Geometry check sheet. Reference: the model listing, model coordinates, mm. A direction names the side the tool comes from. Round coordinates to 2 decimals unless told otherwise and drop trailing zeros. Loops run counter-clockwise (first coordinate to the right, second up) from the corner with the lowest first, then second, coordinate; pieces in that order, holes last. Notation, with made-up numbers: (50.25, -34.75) - (96.25, -34.75) arc R20 ccw to (96.25, -17.75) - close; hole circle Ø5 at (-30, 53). An arc over 180 degrees is marked (long way). Answer as CSV lines item,"result". Start each with the question number.
1) Depth check by flat-ended pin: P1, Ø12, axis at x = 28, z = 6.5, coming from the -Y side; P2, Ø6, axis at x = 10, z = 10.5, coming from the +Y side; P3, Ø8, axis at y = 27.5, z = 10, coming from the +X side. Enter the tip coordinate at first touch or a pass-through.
2) Cross-section at C-C on x = 10. Record the boundary of the cut face in (y, z), and give its area (3 significant figures).
3) Draft check along Z on faces 1 (the cylindrical face through (14.77, 29.89, 9)), 2 (the flat face through (19, 0, 10)), 3 (the flat face through (19, 17, 21)). Enter one of: released by +Z, released by -Z, zero draft, split by the parting line, or undercut.
4) Cross-section at B-B on y = 21. Record the boundary of the cut face in (x, z).
5) Thickness scan on line 1 along X through (y, z) = (29.3, 10.5); line 2 along Z through (x, y) = (10, 7); line 3 along Y through (x, z) = (26, 20). Record the ranges inside material, lowest first.
6) Cross-section at A-A on z = 10.5. Record the boundary of the cut face in (x, y).
7) Cross-section at D-D on z = 4.75. Record the boundary of the cut face in (x, y), and give its area (3 significant figures).
8) Access from +Z, -Z, +X, -X, +Y, -Y to the whole of each face (thin tool, end or side, straight path). Record for faces 4 (the cylindrical face through (7.897, 13.837, 12.112)), 5 (the flat face through (30, 20, 10)), 6 (the flat face through (12, 27, 13)), 7 (the flat face through (32, 28, 10)).
from build123d import *

# Parameters (mm, degrees)
BOSS_EXTRUDE1_DEPTH = 21
SKETCH2_R           = 2.65
CUT_EXTRUDE1_DEPTH  = 34
SKETCH3_R           = 5
CUT_EXTRUDE2_DEPTH  = 6
FILLET1_R           = 0.3


with BuildPart() as part:
    # Sketch1 → Boss-Extrude1 (new body)
    with BuildSketch(Plane.XY):
        Polygon((32, 33), (32, 22.2), (24, 22.2), (24, 20), (37, 20), (37, 0), (0, 0), (0, 33), align=None)
    extrude(amount=BOSS_EXTRUDE1_DEPTH)

    # Sketch2 → Cut-Extrude1 (cut, through all)
    with BuildSketch(Plane(origin=(0, 33, 0), x_dir=(1, 0, 0), z_dir=(0, 1, 0))):
        with Locations((10, -10.5)):
            Circle(SKETCH2_R)
    extrude(amount=-CUT_EXTRUDE1_DEPTH, mode=Mode.SUBTRACT)

    # Sketch3 → Cut-Extrude2 (cut)
    with BuildSketch(Plane(origin=(0, 33, 0), x_dir=(1, 0, 0), z_dir=(0, 1, 0))):
        with Locations((10, -10.5)):
            Circle(SKETCH3_R)
    extrude(amount=-CUT_EXTRUDE2_DEPTH, mode=Mode.SUBTRACT)

    # Fillet1
    fillet1_edges = [part.edges().sort_by_distance(p)[0] for p in [
        (30.5, 20, 0),
        (37, 10, 0),
        (18.5, 0, 0),
        (0, 16.5, 0),
        (37, 10, 21),
        (0, 33, 10.5),
        (32, 33, 10.5),
        (32, 22.2, 10.5),
        (24, 22.2, 10.5),
        (24, 20, 10.5),
        (37, 20, 10.5),
        (37, 0, 10.5),
        (0, 0, 10.5),
        (30.5, 20, 21),
        (24, 21.1, 21),
        (28, 22.2, 21),
        (7.35, 0, 10.5),
        (32, 27.6, 21),
        (5, 33, 10.5),
        (16, 33, 21),
        (0, 16.5, 21),
        (16, 33, 0),
        (18.5, 0, 21),
        (32, 27.6, 0),
        (28, 22.2, 0),
        (24, 21.1, 0),
    ]]
    fillet(fillet1_edges, radius=FILLET1_R)


solid = part.part
Answer block:
1,P1,"stops at y = 0"
1,P2,"stops at y = 27"
1,P3,"stops at x = 32"
2,outline,"(0, 0.3) arc R0.3 ccw to (0.3, 0) - (32.7, 0) arc R0.3 ccw to (33, 0.3) - (33, 5.2) arc R0.3 ccw to (32.7, 5.5) - (27, 5.5) - (27, 7.85) - (0.3, 7.85) arc R0.3 ccw to (0, 7.55) - close; (0, 13.45) arc R0.3 ccw to (0.3, 13.15) - (27, 13.15) - (27, 15.5) - (32.7, 15.5) arc R0.3 ccw to (33, 15.8) - (33, 20.7) arc R0.3 ccw to (32.7, 21) - (0.3, 21) arc R0.3 ccw to (0, 20.7) - close"
2,area,"490 mm^2"
3,face 1,"undercut"
3,face 2,"zero draft"
3,face 3,"released by +Z"
4,outline,"(0, 0.3) arc R0.3 ccw to (0.3, 0) - (23.7, 0) arc R0.3 ccw to (24, 0.3) - (24, 20.7) arc R0.3 ccw to (23.7, 21) - (0.3, 21) arc R0.3 ccw to (0, 20.7) - close; hole circle Ø5.3 at (10, 10.5)"
5,line 1,"x = 0 to 5, 15 to 32"
5,line 2,"z = 0 to 7.85, 13.15 to 21"
5,line 3,"y = 0 to 20, 22.2 to 33"
6,outline,"(0, 0.3) arc R0.3 ccw to (0.3, 0) - (7.05, 0) arc R0.3 ccw to (7.35, 0.3) - (7.35, 27) - (5, 27) - (5, 32.7) arc R0.3 ccw to (4.7, 33) - (0.3, 33) arc R0.3 ccw to (0, 32.7) - close; (12.65, 0.3) arc R0.3 ccw to (12.95, 0) - (36.7, 0) arc R0.3 ccw to (37, 0.3) - (37, 19.7) arc R0.3 ccw to (36.7, 20) - (24.3, 20) arc R0.3 cw to (24, 20.3) - (24, 21.9) arc R0.3 cw to (24.3, 22.2) - (31.7, 22.2) arc R0.3 ccw to (32, 22.5) - (32, 32.7) arc R0.3 ccw to (31.7, 33) - (15.3, 33) arc R0.3 ccw to (15, 32.7) - (15, 27) - (12.65, 27) - close"
7,outline,"(0, 0.3) arc R0.3 ccw to (0.3, 0) - (36.7, 0) arc R0.3 ccw to (37, 0.3) - (37, 19.7) arc R0.3 ccw to (36.7, 20) - (24.3, 20) arc R0.3 cw to (24, 20.3) - (24, 21.9) arc R0.3 cw to (24.3, 22.2) - (31.7, 22.2) arc R0.3 ccw to (32, 22.5) - (32, 32.7) arc R0.3 ccw to (31.7, 33) - (0.3, 33) arc R0.3 ccw to (0, 32.7) - close"
7,area,"1,140 mm^2"
8,face 4,"+Y, -Y"
8,face 5,"+Z, -Z, +X"
8,face 6,"+Y"
8,face 7,"+Z, -Z, +X, +Y"
